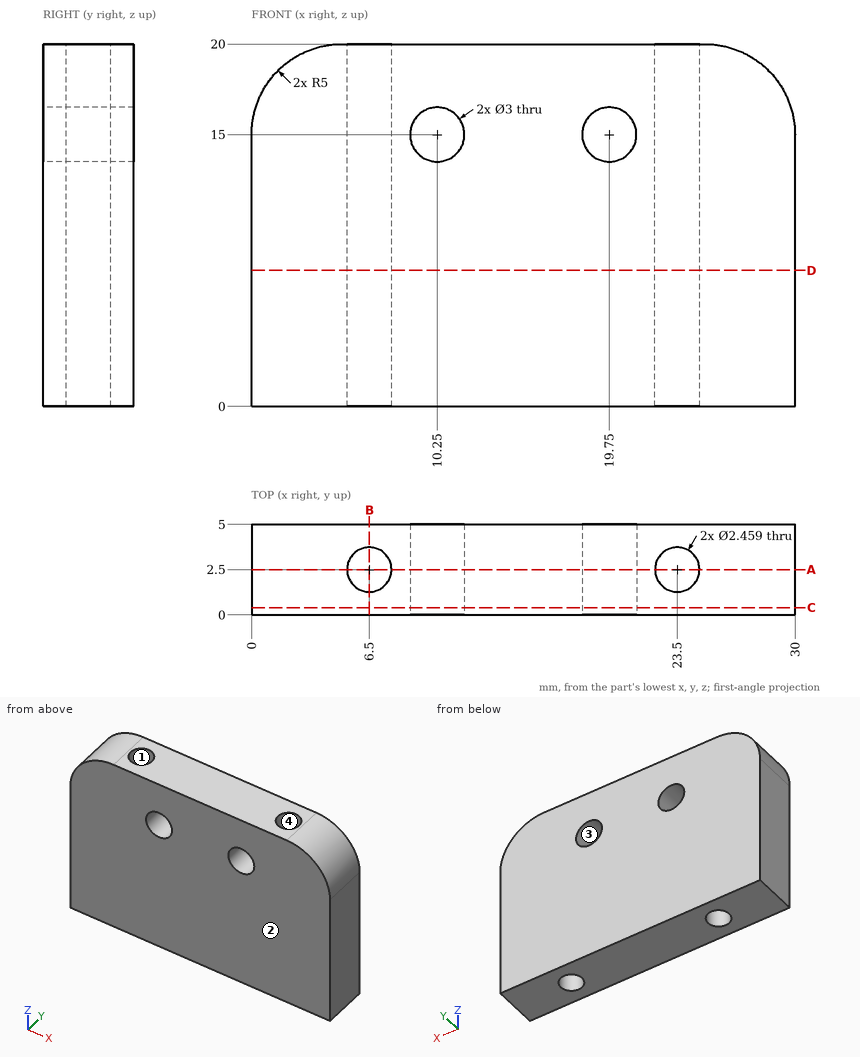
Geometry check sheet. Reference: drawing and pictorial views, mm from the part's lowest x, y, z. Round coordinates to 2 decimals unless told otherwise and drop trailing zeros. Write each loop counter-clockwise with the first axis right and the second up, starting at its lowest first coordinate (ties: lowest second). Pieces come first, ordered by that corner, then holes.
(1) Section check B-B (x = 6.5). Enter the section's corners in (y, z), plus the area to 3 significant figures.
Returned:
outline: (0, 0) - (1.27, 0) - (1.27, 20) - (0, 20) - close; (3.73, 0) - (5, 0) - (5, 20) - (3.73, 20) - close
area: 50.8 mm2
(2) Mould release check, pull along Y, two halves, no side actions. Record for the marked faces 1, 2, 3 and 4: pulls with the +Y half, pulls with the -Y half, needs draft (parallel to the pull), parting line crosses it, or undercut.
Returned:
face 1: undercut
face 2: pulls with the -Y half
face 3: needs draft
face 4: undercut
(3) Section check A-A (y = 2.5). Enter the section's corners in (x, z), plus the area to 3 significant figures.
Returned:
outline: (0, 0) - (5.27, 0) - (5.27, 20) - (5, 20) arc R5 ccw to (0, 15) - close; (7.73, 0) - (22.27, 0) - (22.27, 20) - (7.73, 20) - close; (24.73, 0) - (30, 0) - (30, 15) arc R5 ccw to (25, 20) - (24.73, 20) - close; hole circle Ø3 at (10.25, 15); hole circle Ø3 at (19.75, 15)
area: 477 mm2
(4) Material ranges on line 1 (Z direction, x = 10.25, y = 1.5); line 2 (X direction, y = 2.85, z = 15); line 3 (X direction, y = 0.45, z = 13.75), recorded low to high.
Returned:
line 1: z = 0 to 13.5, 16.5 to 20
line 2: x = 0 to 5.32, 7.68 to 8.75, 11.75 to 18.25, 21.25 to 22.32, 24.68 to 30
line 3: x = 0 to 9.42, 11.08 to 18.92, 20.58 to 30
(5) Section check C-C (y = 0.4). Enter the section's corners in (x, z).
Returned:
outline: (0, 0) - (30, 0) - (30, 15) arc R5 ccw to (25, 20) - (5, 20) arc R5 ccw to (0, 15) - close; hole circle Ø3 at (10.25, 15); hole circle Ø3 at (19.75, 15)
(6) Section check D-D (z = 7.5). Enter the section's corners in (x, y).
Returned:
outline: (0, 0) - (30, 0) - (30, 5) - (0, 5) - close; hole circle Ø2.46 at (6.5, 2.5); hole circle Ø2.46 at (23.5, 2.5)
